```python
from build123d import *

# Parameters (mm, degrees)
SKETCH1_R           = 28.5
SKETCH1_R_2         = 19.5
BOSS_EXTRUDE1_DEPTH = 2
SKETCH2_R           = 27.5
SKETCH2_R_2         = 19.5
BOSS_EXTRUDE2_DEPTH = 4.5
SKETCH3_R           = 1.25
CUT_EXTRUDE1_DEPTH  = 41.825849654
CIRPATTERN1_COUNT   = 6
SKETCH5_R           = 19.5
SKETCH5_R_2         = 16.5
BOSS_EXTRUDE3_DEPTH = 6.5
SKETCH6_R           = 1.25
CUT_EXTRUDE2_DEPTH  = 10
CIRPATTERN2_COUNT   = 3
SKETCH8_R           = 3
CUT_EXTRUDE4_DEPTH  = 3.5
CIRPATTERN4_COUNT   = 3
SKETCH9_R           = 1.5
CUT_EXTRUDE5_DEPTH  = 41.456767048


with BuildPart() as part:
    # Sketch1 → Boss-Extrude1 (new body)
    with BuildSketch(Plane.XY):
        Circle(SKETCH1_R)
        Circle(SKETCH1_R_2, mode=Mode.SUBTRACT)
    extrude(amount=BOSS_EXTRUDE1_DEPTH)

    # Sketch2 → Boss-Extrude2 (add)
    with BuildSketch(Plane.XY.offset(2)):
        Circle(SKETCH2_R)
        Circle(SKETCH2_R_2, mode=Mode.SUBTRACT)
    extrude(amount=BOSS_EXTRUDE2_DEPTH)

    # Sketch3 → Cut-Extrude1 (cut, through all)
    with BuildSketch(Plane.XY.offset(6.5)):
        with Locations((0, 24)):
            Circle(SKETCH3_R)
    cut_extrude1 = extrude(amount=-CUT_EXTRUDE1_DEPTH, mode=Mode.SUBTRACT)

    # CirPattern1: Cut-Extrude1 ×6 about axis
    cirpattern1_axis = Axis((0, 0, 0), (0, 0, 1))
    for i in range(1, CIRPATTERN1_COUNT):
        add(cut_extrude1.rotate(cirpattern1_axis, i * 360 / CIRPATTERN1_COUNT), mode=Mode.SUBTRACT)

    # Sketch5 → Boss-Extrude3 (add)
    with BuildSketch(Plane(origin=(0, 0, 0), x_dir=(-1, 0, 0), z_dir=(0, 0, -1))):
        Circle(SKETCH5_R)
        Circle(SKETCH5_R_2, mode=Mode.SUBTRACT)
    extrude(amount=-BOSS_EXTRUDE3_DEPTH)

    # Sketch6 → Cut-Extrude2 (cut)
    with BuildSketch(Plane(origin=(0, 0, 0), x_dir=(-1, 0, 0), z_dir=(0, 0, -1))):
        with Locations((10, 17.320508076)):
            Circle(SKETCH6_R)
    cut_extrude2 = extrude(amount=-CUT_EXTRUDE2_DEPTH, mode=Mode.SUBTRACT)

    # CirPattern2: Cut-Extrude2 ×3 about axis
    cirpattern2_axis = Axis((0, 0, 0), (0, 0, 1))
    for i in range(1, CIRPATTERN2_COUNT):
        add(cut_extrude2.rotate(cirpattern2_axis, i * 360 / CIRPATTERN2_COUNT), mode=Mode.SUBTRACT)

    # Sketch8 → Cut-Extrude4 (cut)
    with BuildSketch(Plane(origin=(0, 0, 0), x_dir=(-1, 0, 0), z_dir=(0, 0, -1))):
        with Locations((0, 24)):
            Circle(SKETCH8_R)
    cut_extrude4 = extrude(amount=-CUT_EXTRUDE4_DEPTH, mode=Mode.SUBTRACT)

    # CirPattern4: Cut-Extrude4 ×3 about axis
    cirpattern4_axis = Axis((0, 0, 0), (0, 0, 1))
    for i in range(1, CIRPATTERN4_COUNT):
        add(cut_extrude4.rotate(cirpattern4_axis, i * 360 / CIRPATTERN4_COUNT), mode=Mode.SUBTRACT)

    # Sketch9 → Cut-Extrude5 (cut, through all)
    with BuildSketch(Plane(origin=(0, 0, 3.5), x_dir=(-1, 0, 0), z_dir=(0, 0, -1))):
        with Locations((0, 24)):
            Circle(SKETCH9_R)
        with Locations((20.784609691, -12)):
            Circle(SKETCH9_R)
        with Locations((-20.784609691, -12)):
            Circle(SKETCH9_R)
    extrude(amount=-CUT_EXTRUDE5_DEPTH, mode=Mode.SUBTRACT)


solid = part.part
```
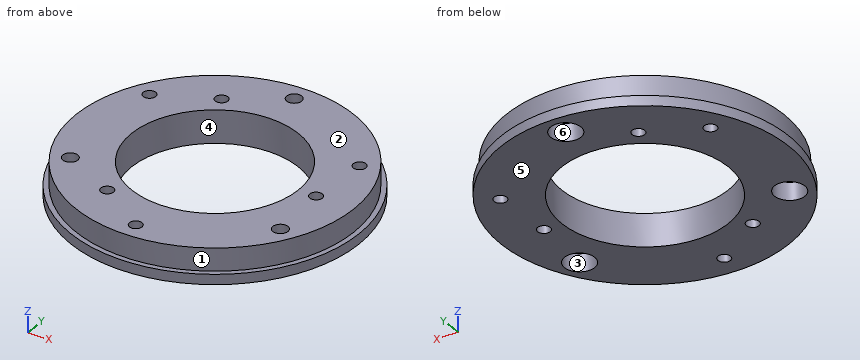
Input: part model. Units: mm. Frame: model coordinates. Face numbers are marked on the shaded views. A direction names the side the tool comes from. Round coordinates to 2 decimals unless told otherwise and drop trailing zeros. Loops run counter-clockwise (first coordinate to the right, second up) from the corner with the lowest first, then second, coordinate; pieces in that order, holes last. Notation, with made-up numbers: M 44.25,29 L 52.25,29 A14 ccw 52.25,50 Z; hole C -5.75,-2.75 d4. An arc over 180 degrees is marked long. Answer in a Markdown table with one row per item. Add a question column.
1. Section B-B (x = 0). Output: boundary loops of the cut face in (y, z), and give its area (3 significant figures).
2. Contact query for flat-ended pins moving along their axis: pin 1 (1.8 mm diameter, centred on x = -0.5, y = 24.5, fed in from -Z); pin 2 (2 mm diameter, centred on x = 20.78, y = 12, fed in from -Z); pin 3 (2 mm diameter, centred on x = 3.5, z = 3.5, fed in from +Y); pin 4 (1.5 mm diameter, centred on y = 19, z = 2.5, fed in from -X). Output: stop coordinate, or through.
3. Section A-A (y = 0). Output: boundary loops of the cut face in (x, z), and give its area (3 significant figures).
4. Set-up query: the marked faces 5 and 6. Return all of +Z, -Z, +X, -X, +Y, -Y with unobstructed straight access to the full face (end or side cutting, diameter ignored); none if empty.
5. Section C-C (y = 24). Output: boundary loops of the cut face in (x, z), and give its area (3 significant figures).
6. Section D-D (x = 14). Output: boundary loops of the cut face in (y, z).
7. Mould query, pull axis X, two halves, no side actions, for the marked faces 1, 2, 3 and 4. Classes: released by +X, released by -X, zero draft, split by the parting line, or undercut.
8. Ray query, probe 1 along Y at (x, z) = (0, 3.25); probe 2 along Y at (x, z) = (2.5, 1.5); probe 3 along Y at (x, z) = (-10, 5). Return the intervals inside material, ascending.
Values follow:
| question | item | result |
|---|---|---|
| 1 | outline | M -28.5,0 L -25.25,0 L -25.25,6.5 L -27.5,6.5 L -27.5,2 L -28.5,2 Z; M -22.75,0 L -16.5,0 L -16.5,6.5 L -22.75,6.5 Z; M 16.5,0 L 21,0 L 21,3.5 L 22.5,3.5 L 22.5,6.5 L 16.5,6.5 Z; M 25.5,3.5 L 27,3.5 L 27,0 L 28.5,0 L 28.5,2 L 27.5,2 L 27.5,6.5 L 25.5,6.5 Z |
| 1 | area | 101 mm^2 |
| 2 | pin 1 | z = 3.5 |
| 2 | pin 2 | through |
| 2 | pin 3 | y = 27.39 |
| 2 | pin 4 | x = -21.73 |
| 3 | outline | M -28.5,0 L -16.5,0 L -16.5,6.5 L -27.5,6.5 L -27.5,2 L -28.5,2 Z; M 16.5,0 L 18.75,0 L 18.75,6.5 L 16.5,6.5 Z; M 21.25,0 L 28.5,0 L 28.5,2 L 27.5,2 L 27.5,6.5 L 21.25,6.5 Z |
| 3 | area | 131 mm^2 |
| 4 | face 5 | -Z, +X, -X, +Y, -Y |
| 4 | face 6 | -Z |
| 5 | outline | M -15.37,0 L -3,0 L -3,3.5 L -1.5,3.5 L -1.5,6.5 L -13.43,6.5 L -13.43,2 L -15.37,2 Z; M 1.5,3.5 L 3,3.5 L 3,0 L 15.37,0 L 15.37,2 L 13.43,2 L 13.43,6.5 L 1.5,6.5 Z |
| 5 | area | 152 mm^2 |
| 6 | outline | M -24.82,0 L -8.73,0 L -8.73,6.5 L -23.67,6.5 L -23.67,2 L -24.82,2 Z; M 8.73,0 L 24.82,0 L 24.82,2 L 23.67,2 L 23.67,6.5 L 8.73,6.5 Z |
| 7 | face 1 | split by the parting line |
| 7 | face 2 | zero draft |
| 7 | face 3 | undercut |
| 7 | face 4 | undercut |
| 8 | probe 1 | -27.5 to -25.25, -22.75 to -16.5, 16.5 to 21, 27 to 27.5 |
| 8 | probe 2 | -28.39 to -16.31, 16.31 to 22.34, 25.66 to 28.39 |
| 8 | probe 3 | -25.62 to -18.57, -16.07 to -13.12, 13.12 to 16.07, 18.57 to 25.62 |
